Answer from the drawing. Dimensions are ordinates in mm from the lowest x, y and z of the part. A direction names the side the tool comes from. Give positions to 0.01 mm unless a question says otherwise; leave off trailing zeros. Loops run counter-clockwise (first coordinate to the right, second up) from the corner with the lowest first, then second, coordinate; pieces in that order, holes last. Notation, with made-up numbers: M 33.5,11 L 66.5,11 A29 cw 66.5,36 Z; hole C -8,56.5 d3. An arc over 180 degrees is marked long. Use a Markdown table: item, result.
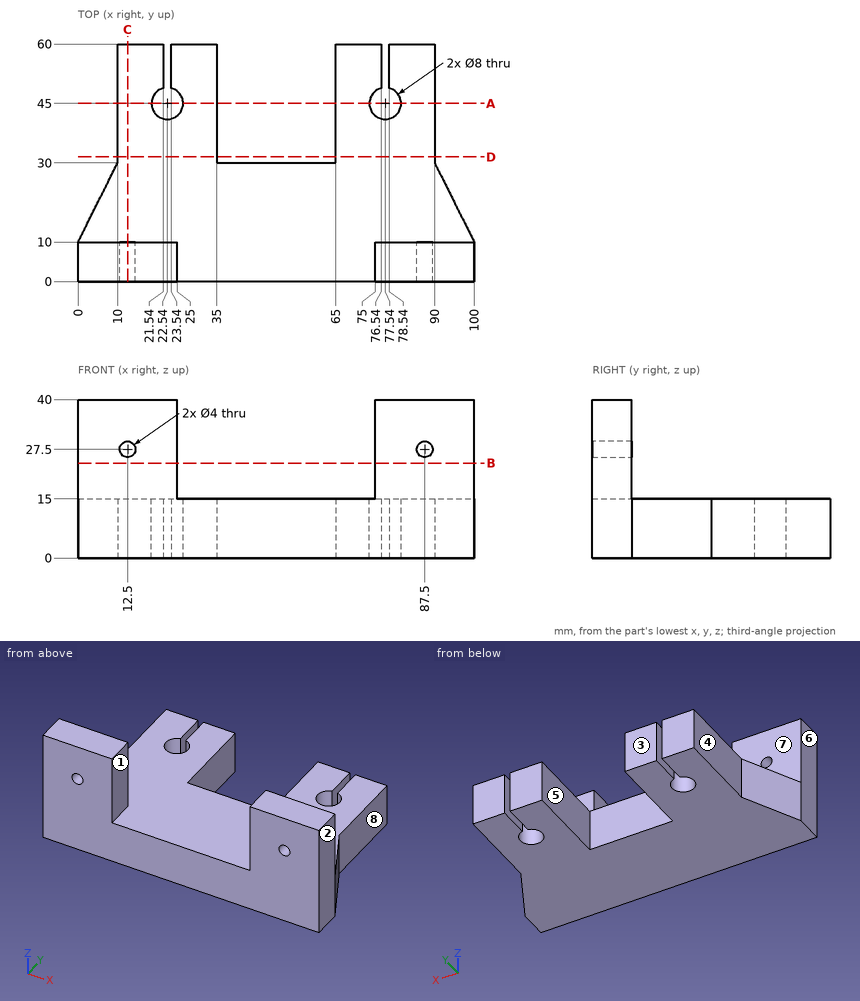
(1) Which of the six approach directions +Z, -Z, +X, -X, +Y, -Y give full straight-line access (tool end or side, diameter ignored) to the marked faces 5, 6, 7 and 8?
Entries:
| item | result |
|---|---|
| face 5 | +Z, -Z, +Y |
| face 6 | +Z, -Z, -X, +Y, -Y |
| face 7 | +Z, +X, -X, +Y |
| face 8 | +Z, -Z, +X, +Y |
(2) Consider probe 1 along X at (y, z) = (45, 5.5); probe 2 along X at (y, z) = (4.75, 27.5); probe 3 along Z at (x, y) = (9.5, 27.5). Determine where each line is inside the solid, lowest interval first. Write a range as [from, to].
Entries:
| item | result |
|---|---|
| probe 1 | x = [10, 18.54], [26.54, 35], [65, 73.54], [81.54, 90] |
| probe 2 | x = [0, 10.5], [14.5, 25], [75, 85.5], [89.5, 100] |
| probe 3 | z = [0, 15] |
(3) A cutting plane is placed at B-B (z = 24). Write down the section's boundary in (x, y).
Entries:
| item | result |
|---|---|
| outline | M 0,0 L 25,0 L 25,10 L 0,10 Z; M 75,0 L 100,0 L 100,10 L 75,10 Z |
(4) A cutting plane is placed at D-D (y = 31.5). Write down the section's boundary in (x, z).
Entries:
| item | result |
|---|---|
| outline | M 10,0 L 35,0 L 35,15 L 10,15 Z; M 65,0 L 90,0 L 90,15 L 65,15 Z |
(5) The mould has two halves that part along X. Classify the marked faces 1, 2, 3 and 4: released by +X, released by -X, zero draft, split by the parting line, or undercut.
Entries:
| item | result |
|---|---|
| face 1 | undercut |
| face 2 | released by +X |
| face 3 | zero draft |
| face 4 | released by -X |
(6) A cutting plane is placed at C-C (x = 12.5). Write down the section's boundary in (y, z), and give its area (3 significant figures).
Entries:
| item | result |
|---|---|
| outline | M 0,0 L 60,0 L 60,15 L 10,15 L 10,25.5 L 0,25.5 Z; M 0,29.5 L 10,29.5 L 10,40 L 0,40 Z |
| area | 1,110 mm² |
(7) A cutting plane is placed at A-A (y = 45). Write down the section's boundary in (x, z).
Entries:
| item | result |
|---|---|
| outline | M 10,0 L 18.54,0 L 18.54,15 L 10,15 Z; M 26.54,0 L 35,0 L 35,15 L 26.54,15 Z; M 65,0 L 73.54,0 L 73.54,15 L 65,15 Z; M 81.54,0 L 90,0 L 90,15 L 81.54,15 Z |
(8) Given P1, Ø7.5, axis at y = 44.5, z = 4, coming from the -X side; P2, Ø12, axis at x = 27.5, y = 48, coming from the +Z side; P3, Ø12, axis at y = 48, z = 4.5, coming from the +X side; P4, Ø7, axis at x = 22.54, y = 45, coming from the -Z side, each flat-ended and moving along its own axis, determine where each tip first touches the part or whether it passes through.
Entries:
| item | result |
|---|---|
| P1 | stops at x = 10 |
| P2 | stops at z = 15 |
| P3 | stops at x = 90 |
| P4 | passes through |
